Geometry: final body of the model. Coordinates: model frame, mm. A direction names the side the tool comes from. Give positions to 0.01 mm unless a question says otherwise; leave off trailing zeros. Write each loop counter-clockwise with the first axis right and the second up, starting at its lowest first coordinate (ties: lowest second). Pieces come first, ordered by that corner, then holes. Notation, with made-up numbers: M 49.5,-7.5 L 93.5,-7.5 A25 cw 93.5,5.5 Z; hole C -28.5,-1 d9. An arc over 180 degrees is marked long. Use a Markdown table: item, result. Add a question column.
(1) Cut plane D-D (x = -56). Output: boundary loops of the cut face in (y, z), plus the area to 3 significant figures.
(2) Draft query along Z for faces 1 (the flat face through (49.7, 35.2, 122.5)), 2 (the flat face through (19, 41, 124.5)), 3 (the flat face through (38, 0, 29.5)). Return one class per face: released by +Z, released by -Z, zero draft, split by the parting line, or undercut.
(3) Pin query (flat end, axial travel): pin 1 Ø2 at (y, z) = (-19.5, 78.5) entering from +X; pin 2 Ø6.5 at (x, y) = (-41, -46.5) entering from +Z; pin 3 Ø1.5 at (y, z) = (-24.5, 33) entering from -X. Return the tip coordinate at first contact, or that it passes through.
(4) Cut plane B-B (x = -25). Output: boundary loops of the cut face in (y, z), plus the area to 3 significant figures.
(5) Cut plane A-A (y = 34). Output: boundary loops of the cut face in (x, z), plus the area to 3 significant figures.
(6) Cut plane C-C (z = 54.5). Output: boundary loops of the cut face in (x, y), plus the area to 3 significant figures.
(7) Reachability of faces 4 (the flat face through (38, 20, 54)), 5 (the flat face through (45, 10, 115)), 6 (the flat face through (43, -3, 59)) from +Z, -Z, +X, -X, +Y, -Y: full face, straight path, thin tool, end or side. Return the list, or none.
(8) Material intervals for L1, parallel to Y at x = -43.5, z = 87.9; L2, parallel to Y at x = 37.5, z = 36; L3, parallel to Y at x = -32.5, z = 116, sorted ascending.
```python
from build123d import *

# Parameters (mm, degrees)
SKETCH1_W                = 85
SKETCH1_H                = 95
BOSS_EXTRUDE1_DEPTH      = 4.5
SKETCH2_W                = 4.5
SKETCH2_H                = 85
BOSS_EXTRUDE2_DEPTH      = 120
SKETCH3_W                = 90.5
SKETCH3_H                = 4.5
BOSS_EXTRUDE3_DEPTH      = 120
CUT_EXTRUDE1_REACH       = 141.867
SKETCH4_R                = 22.5
CUT_EXTRUDE3_DEPTH       = 163.269837
SKETCH8_W                = 2.25
SKETCH8_H                = 2
CUT_EXTRUDE4_DEPTH       = 90.5
SKETCH9_W                = 85
SKETCH9_H                = 4.5
BOSS_EXTRUDE5_DEPTH      = 4.5
SKETCH11_W               = 40
SKETCH11_H               = 50
BOSS_EXTRUDE7_DEPTH      = 10
SKETCH12_W               = 30.5
SKETCH12_H               = 40.5
CUT_EXTRUDE5_DEPTH       = 10
SKETCH13_R               = 5
CUT_EXTRUDE6_DEPTH       = 163.269837
SKETCH14_W               = 8
SKETCH14_H               = 2
BOSS_EXTRUDE8_DEPTH      = 8
CUT_EXTRUDE8_DEPTH       = 143.782176759
CUT_EXTRUDE8_DEPTH_BACK  = 143.782176759
SKETCH16_R               = 1.7
SKETCH17_W               = 8
SKETCH17_H               = 2
BOSS_EXTRUDE9_DEPTH      = 8
CUT_EXTRUDE9_DEPTH       = 143.443848586
CUT_EXTRUDE9_DEPTH_BACK  = 143.443848586
SKETCH18_R               = 1.7
SKETCH19_W               = 2.25
SKETCH19_H               = 2
BOSS_EXTRUDE10_DEPTH     = 4.5
SKETCH20_W               = 8
SKETCH20_H               = 2
BOSS_EXTRUDE11_DEPTH     = 8
SKETCH22_W               = 8
SKETCH22_H               = 2
BOSS_EXTRUDE12_DEPTH     = 8
CUT_EXTRUDE10_DEPTH      = 119.80998485
CUT_EXTRUDE10_DEPTH_BACK = 119.80998485
SKETCH21_R               = 1.7
FILLET2_R                = 2
FILLET3_R                = 1
CUT_EXTRUDE11_DEPTH      = 170.291169291
CUT_EXTRUDE11_DEPTH_BACK = 170.291169291


with BuildPart() as part:
    # Sketch1 → Boss-Extrude1 (new body)
    with BuildSketch(Plane(origin=(0, 0, 0), x_dir=(0, 1, 0), z_dir=(0, 0, 1))):
        Rectangle(SKETCH1_W, SKETCH1_H)
    extrude(amount=BOSS_EXTRUDE1_DEPTH)

    # Sketch2 → Boss-Extrude2 (add)
    with BuildSketch(Plane.XY.offset(4.5)):
        with Locations((45.25, 0)):
            Rectangle(SKETCH2_W, SKETCH2_H)
    extrude(amount=BOSS_EXTRUDE2_DEPTH)

    # Sketch3 → Boss-Extrude3 (add)
    with BuildSketch(Plane.XY.offset(4.5)):
        with Locations((-2.25, 40.25)):
            Rectangle(SKETCH3_W, SKETCH3_H)
        with Locations((-2.25, -40.25)):
            Rectangle(SKETCH3_W, SKETCH3_H)
    extrude(amount=BOSS_EXTRUDE3_DEPTH)

    # Sketch4 → Cut-Extrude1 (cut, up to next)
    with BuildSketch(Plane(origin=(0, 0, 0), x_dir=(1, 0, 0), z_dir=(0, 0, -1)), mode=Mode.PRIVATE) as cut_extrude1_sk1:
        with Locations(Location((9, 0, 0), (0, 0, 180))):
            Circle(SKETCH4_R)
    cut_extrude1_tool1 = extrude(cut_extrude1_sk1.sketch, amount=-CUT_EXTRUDE1_REACH, mode=Mode.PRIVATE) & part.part
    add(cut_extrude1_tool1.solids().sort_by_distance((9, 0, 0))[0], mode=Mode.SUBTRACT)

    # Sketch7 → Cut-Extrude3 (cut, through all)
    with BuildSketch(Plane(origin=(-47.5, 0, 0), x_dir=(0, -1, 0), z_dir=(-1, 0, 0))):
        Polygon((-38, 85.25), (-40.25, 85.25), (-40.25, 87.25), (-42.5, 87.25), (-42.5, 37.25), (-40.25, 37.25), (-40.25, 39.25), (-38, 39.25), align=None)
        Polygon((40.25, 39.25), (38, 39.25), (38, 85.25), (40.25, 85.25), (40.25, 87.25), (42.5, 87.25), (42.5, 37.25), (40.25, 37.25), align=None)
    extrude(amount=-CUT_EXTRUDE3_DEPTH, mode=Mode.SUBTRACT)

    # Sketch8 → Cut-Extrude4 (cut)
    with BuildSketch(Plane(origin=(-47.5, 0, 0), x_dir=(0, -1, 0), z_dir=(-1, 0, 0))):
        with Locations((-39.125, 123.5)):
            Rectangle(SKETCH8_W, SKETCH8_H)
        with Locations((39.125, 123.5)):
            Rectangle(SKETCH8_W, SKETCH8_H)
    extrude(amount=-CUT_EXTRUDE4_DEPTH, mode=Mode.SUBTRACT)

    # Sketch9 → Boss-Extrude5 (add)
    with BuildSketch(Plane(origin=(-47.5, 0, 0), x_dir=(0, -1, 0), z_dir=(-1, 0, 0))):
        with Locations((0, 2.25)):
            Rectangle(SKETCH9_W, SKETCH9_H)
    extrude(amount=BOSS_EXTRUDE5_DEPTH)

    # Sketch11 → Boss-Extrude7 (add)
    with BuildSketch(Plane(origin=(43, 0, 0), x_dir=(0, -1, 0), z_dir=(-1, 0, 0))):
        with Locations((0, 54.5)):
            Rectangle(SKETCH11_W, SKETCH11_H)
    extrude(amount=BOSS_EXTRUDE7_DEPTH)

    # Sketch12 → Cut-Extrude5 (cut)
    with BuildSketch(Plane(origin=(33, 0, 0), x_dir=(0, -1, 0), z_dir=(-1, 0, 0))):
        with Locations((0, 54.5)):
            Rectangle(SKETCH12_W, SKETCH12_H)
    extrude(amount=-CUT_EXTRUDE5_DEPTH, mode=Mode.SUBTRACT)

    # Sketch13 → Cut-Extrude6 (cut, through all)
    with BuildSketch(Plane(origin=(43, 0, 0), x_dir=(0, -1, 0), z_dir=(-1, 0, 0))):
        with Locations(Location((0, 54.5, 0), (0, 0, 90))):
            Circle(SKETCH13_R)
    extrude(amount=-CUT_EXTRUDE6_DEPTH, mode=Mode.SUBTRACT)

    # Sketch14 → Boss-Extrude8 (add)
    with BuildSketch(Plane.YZ.offset(47.5)):
        with Locations((-34, 123.5)):
            Rectangle(SKETCH14_W, SKETCH14_H)
        with Locations((34, 123.5)):
            Rectangle(SKETCH14_W, SKETCH14_H)
    extrude(amount=BOSS_EXTRUDE8_DEPTH)

    # Sketch16 → Cut-Extrude8 (cut, two sides: drawn at the far end of the back side and taken through both)
    with BuildSketch(Plane.XY.offset(124.5).offset(-CUT_EXTRUDE8_DEPTH_BACK)):
        with Locations((51.5, 34)):
            Circle(SKETCH16_R)
        with Locations((51.5, -34)):
            Circle(SKETCH16_R)
    extrude(amount=CUT_EXTRUDE8_DEPTH + CUT_EXTRUDE8_DEPTH_BACK, mode=Mode.SUBTRACT)

    # Sketch17 → Boss-Extrude9 (add)
    with BuildSketch(Plane(origin=(-52, 0, 0), x_dir=(0, -1, 0), z_dir=(-1, 0, 0))):
        with Locations((-34, 3.5)):
            Rectangle(SKETCH17_W, SKETCH17_H)
        with Locations((34, 3.5)):
            Rectangle(SKETCH17_W, SKETCH17_H)
    extrude(amount=BOSS_EXTRUDE9_DEPTH)

    # Sketch18 → Cut-Extrude9 (cut, two sides: drawn at the far end of the back side and taken through both)
    with BuildSketch(Plane(origin=(0, 0, 2.5), x_dir=(1, 0, 0), z_dir=(0, 0, -1)).offset(-CUT_EXTRUDE9_DEPTH_BACK)):
        with Locations(Location((-56, -34, 0), (0, 0, 180))):
            Circle(SKETCH18_R)
        with Locations(Location((-56, 34, 0), (0, 0, 180))):
            Circle(SKETCH18_R)
    extrude(amount=CUT_EXTRUDE9_DEPTH + CUT_EXTRUDE9_DEPTH_BACK, mode=Mode.SUBTRACT)

    # Sketch19 → Boss-Extrude10 (add)
    with BuildSketch(Plane.YZ.offset(47.5)):
        with Locations((-41.375, 86.25)):
            Rectangle(SKETCH19_W, SKETCH19_H)
        with Locations((-41.375, 38.25)):
            Rectangle(SKETCH19_W, SKETCH19_H)
        with Locations((41.375, 38.25)):
            Rectangle(SKETCH19_W, SKETCH19_H)
        with Locations((41.375, 86.25)):
            Rectangle(SKETCH19_W, SKETCH19_H)
    extrude(amount=-BOSS_EXTRUDE10_DEPTH)

    # Sketch20 → Boss-Extrude11 (add)
    with BuildSketch(Plane(origin=(0, 42.5, 0), x_dir=(-1, 0, 0), z_dir=(0, 1, 0))):
        with Locations((43.5, 36.25)):
            Rectangle(SKETCH20_W, SKETCH20_H)
        with Locations((43.5, 88.25)):
            Rectangle(SKETCH20_W, SKETCH20_H)
    extrude(amount=BOSS_EXTRUDE11_DEPTH)

    # Sketch22 → Boss-Extrude12 (add)
    with BuildSketch(Plane.XZ.offset(42.5)):
        with Locations((-43.5, 36.25)):
            Rectangle(SKETCH22_W, SKETCH22_H)
        with Locations((-43.5, 88.25)):
            Rectangle(SKETCH22_W, SKETCH22_H)
    extrude(amount=BOSS_EXTRUDE12_DEPTH)

    # Sketch21 → Cut-Extrude10 (cut, two sides: drawn at the far end of the back side and taken through both)
    with BuildSketch(Plane(origin=(0, 0, 35.25), x_dir=(1, 0, 0), z_dir=(0, 0, -1)).offset(-CUT_EXTRUDE10_DEPTH_BACK)):
        with Locations(Location((-43.5, -46.5, 0), (0, 0, 180))):
            Circle(SKETCH21_R)
        with Locations(Location((-43.5, 46.5, 0), (0, 0, 180))):
            Circle(SKETCH21_R)
    extrude(amount=CUT_EXTRUDE10_DEPTH + CUT_EXTRUDE10_DEPTH_BACK, mode=Mode.SUBTRACT)

    # Fillet2
    fillet2_edges = [part.edges().sort_by_distance(p)[0] for p in [
        (47.5, -38, 123.5),
        (47.5, -30, 123.5),
        (55.5, -38, 123.5),
        (55.5, -30, 123.5),
        (47.5, 38, 123.5),
        (47.5, 30, 123.5),
        (55.5, 38, 123.5),
        (55.5, 30, 123.5),
        (-52, 38, 3.5),
        (-52, 30, 3.5),
        (-60, 38, 3.5),
        (-60, 30, 3.5),
        (-52, -38, 3.5),
        (-52, -30, 3.5),
        (-60, -38, 3.5),
        (-60, -30, 3.5),
        (-39.5, 42.5, 36.25),
        (-47.5, 50.5, 36.25),
        (-39.5, 50.5, 36.25),
        (-39.5, 42.5, 88.25),
        (-47.5, 50.5, 88.25),
        (-39.5, 50.5, 88.25),
        (-39.5, -42.5, 36.25),
        (-47.5, -50.5, 36.25),
        (-39.5, -50.5, 36.25),
        (-39.5, -42.5, 88.25),
        (-47.5, -50.5, 88.25),
        (-39.5, -50.5, 88.25),
    ]]
    fillet(fillet2_edges, radius=FILLET2_R)

    # Fillet3
    fillet3_edges = [part.edges().sort_by_distance(p)[0] for p in [
        (-47.5, -39.125, 39.25),
        (-47.5, 39.125, 85.25),
        (-47.5, 40.25, 86.25),
        (-47.5, 40.25, 38.25),
        (-47.5, 39.125, 39.25),
        (-47.5, -40.25, 38.25),
        (-47.5, -40.25, 86.25),
        (-47.5, -39.125, 85.25),
    ]]
    fillet(fillet3_edges, radius=FILLET3_R)

    # Sketch23 → Cut-Extrude11 (cut, two sides: drawn at the far end of the back side and taken through both)
    with BuildSketch(Plane(origin=(43, 0, 0), x_dir=(0, -1, 0), z_dir=(-1, 0, 0)).offset(-CUT_EXTRUDE11_DEPTH_BACK)):
        with BuildLine():
            Line((-10, 124.5), (-10, 105.472696854))
            ThreePointArc((-10, 105.472696854), (0, 95.472696854), (10, 105.472696854))
            Line((10, 105.472696854), (10, 124.5))
            Line((10, 124.5), (-10, 124.5))
        make_face()
    extrude(amount=CUT_EXTRUDE11_DEPTH + CUT_EXTRUDE11_DEPTH_BACK, mode=Mode.SUBTRACT)


solid = part.part
```
Answer list:
| question | item | result |
|---|---|---|
| 1 | outline | M -38,2.5 L -35.7,2.5 L -35.7,4.5 L -38,4.5 Z; M -32.3,2.5 L -30,2.5 L -30,4.5 L -32.3,4.5 Z; M 30,2.5 L 32.3,2.5 L 32.3,4.5 L 30,4.5 Z; M 35.7,2.5 L 38,2.5 L 38,4.5 L 35.7,4.5 Z |
| 1 | area | 18.4 mm² |
| 2 | face 1 | released by -Z |
| 2 | face 2 | released by +Z |
| 2 | face 3 | undercut |
| 3 | pin 1 | x = 47.5 |
| 3 | pin 2 | z = 89.25 |
| 3 | pin 3 | x = 43 |
| 4 | outline | M -42.5,0 L 42.5,0 L 42.5,37.25 L 40.25,37.25 L 40.25,39.25 L 38,39.25 L 38,4.5 L -38,4.5 L -38,39.25 L -40.25,39.25 L -40.25,37.25 L -42.5,37.25 Z; M -42.5,87.25 L -40.25,87.25 L -40.25,85.25 L -38,85.25 L -38,122.5 L -40.25,122.5 L -40.25,124.5 L -42.5,124.5 Z; M 38,85.25 L 40.25,85.25 L 40.25,87.25 L 42.5,87.25 L 42.5,124.5 L 40.25,124.5 L 40.25,122.5 L 38,122.5 Z |
| 4 | area | 1,020 mm² |
| 5 | outline | M -60,2.5 L -57.7,2.5 L -57.7,4.5 L -60,4.5 Z; M -54.3,2.5 L -52,2.5 L -52,0 L 47.5,0 L 47.5,122.5 L 49.8,122.5 L 49.8,124.5 L 43,124.5 L 43,4.5 L -54.3,4.5 Z; M 53.2,122.5 L 55.5,122.5 L 55.5,124.5 L 53.2,124.5 Z |
| 5 | area | 1,010 mm² |
| 6 | outline | M 33,-20 L 43,-20 L 43,-38 L 47.5,-38 L 47.5,-5 L 43,-5 L 43,-15.25 L 33,-15.25 Z; M 33,15.25 L 43,15.25 L 43,5 L 47.5,5 L 47.5,38 L 43,38 L 43,20 L 33,20 Z |
| 6 | area | 392 mm² |
| 7 | face 4 | +Z, -X |
| 7 | face 5 | +Z, +X, -X |
| 7 | face 6 | -X |
| 8 | L1 | -50.5 to -48.2, -44.8 to -38, 38 to 44.8, 48.2 to 50.5 |
| 8 | L2 | -42.5 to -38, -20 to -15.25, 15.25 to 20, 38 to 42.5 |
| 8 | L3 | -42.5 to -38, 38 to 42.5 |
